```python
from build123d import *

# Parameters (mm, degrees)
F0_R     = 29.0195
F1_DEPTH = 19.05
F2_R     = 2.286
F2_R_2   = 29.0195
F2_R_3   = 21.59
F3_DEPTH = 12.7
F5_DEPTH = 3.175


with BuildPart() as f1:
    # F0 (on Top) → F1 (new body)
    with BuildSketch(Plane.XY):
        with BuildLine():
            Line((58.7375, 1.8415), (58.7375, 93.218))
            ThreePointArc((58.7375, 93.218), (0, 151.9555), (-58.7375, 93.218))
            Line((-58.7375, 93.218), (-58.7375, 1.8415))
            ThreePointArc((-58.7375, 1.8415), (-53.848048, -21.620845), (-39.993711, -41.177066))
            ThreePointArc((-39.993711, -41.177066), (-36.998179, -45.405437), (-35.941, -50.478377))
            Line((-35.941, -50.478377), (-35.941, -74.676))
            ThreePointArc((-35.941, -74.676), (-34.081128, -79.166128), (-29.591, -81.026))
            Line((-29.591, -81.026), (29.591, -81.026))
            ThreePointArc((29.591, -81.026), (34.081128, -79.166128), (35.941, -74.676))
            Line((35.941, -74.676), (35.941, -50.478377))
            ThreePointArc((35.941, -50.478377), (36.998179, -45.405437), (39.993711, -41.177066))
            ThreePointArc((39.993711, -41.177066), (53.848048, -21.620845), (58.7375, 1.8415))
        make_face()
        with BuildLine():
            ThreePointArc((-23.241, -37.899), (-39.933751, -21.065855), (-46.0375, 1.8415))
            Line((-46.0375, 1.8415), (-46.0375, 38.162218))
            ThreePointArc((-46.0375, 38.162218), (-43.247692, 44.89741), (-36.5125, 47.687218))
            Line((-36.5125, 47.687218), (36.5125, 47.687218))
            ThreePointArc((36.5125, 47.687218), (43.247692, 44.89741), (46.0375, 38.162218))
            Line((46.0375, 38.162218), (46.0375, 1.8415))
            ThreePointArc((46.0375, 1.8415), (39.933751, -21.065855), (23.241, -37.899))
            Line((23.241, -37.899), (23.241, -68.326))
            Line((23.241, -68.326), (-23.241, -68.326))
            Line((-23.241, -68.326), (-23.241, -37.899))
        make_face(mode=Mode.SUBTRACT)
        with Locations((0, 93.218)):
            Circle(F0_R, mode=Mode.SUBTRACT)
    extrude(amount=F1_DEPTH)

    # F2 (on face) → F3 (join)
    with BuildSketch(Plane(origin=(0, 0, 0), x_dir=(1, 0, 0), z_dir=(0, 0, -1))):
        with BuildLine():
            ThreePointArc((-58.7375, -93.218), (0, -151.9555), (58.7375, -93.218))
            Line((58.7375, -93.218), (58.7375, -1.8415))
            ThreePointArc((58.7375, -1.8415), (53.848048, 21.620845), (39.993711, 41.177066))
            ThreePointArc((39.993711, 41.177066), (36.998179, 45.405437), (35.941, 50.478377))
            Line((35.941, 50.478377), (35.941, 74.676))
            ThreePointArc((35.941, 74.676), (34.081128, 79.166128), (29.591, 81.026))
            Line((29.591, 81.026), (-29.591, 81.026))
            ThreePointArc((-29.591, 81.026), (-34.081128, 79.166128), (-35.941, 74.676))
            Line((-35.941, 74.676), (-35.941, 50.478377))
            ThreePointArc((-35.941, 50.478377), (-36.998179, 45.405437), (-39.993711, 41.177066))
            ThreePointArc((-39.993711, 41.177066), (-53.848048, 21.620845), (-58.7375, -1.8415))
            Line((-58.7375, -1.8415), (-58.7375, -93.218))
        make_face()
        with Locations((-32.7025, -36.765218)):
            Circle(F2_R, mode=Mode.SUBTRACT)
        with Locations((0, -93.218)):
            Circle(F2_R_2, mode=Mode.SUBTRACT)
        with Locations((32.7025, -36.765218)):
            Circle(F2_R, mode=Mode.SUBTRACT)
        Circle(F2_R_3, mode=Mode.SUBTRACT)
        with Locations((0, 35.56)):
            Circle(F2_R, mode=Mode.SUBTRACT)
    extrude(amount=-F3_DEPTH)

    # F4 (on face) → F5 (cut)
    with BuildSketch(Plane.XY):
        with BuildLine():
            ThreePointArc((-52.3875, 1.8415), (-48.026637, -19.084375), (-35.670066, -36.52641))
            ThreePointArc((-35.670066, -36.52641), (-31.176768, -42.868968), (-29.591, -50.478377))
            Line((-29.591, -50.478377), (-29.591, -74.676))
            Line((-29.591, -74.676), (29.591, -74.676))
            Line((29.591, -74.676), (29.591, -50.478377))
            ThreePointArc((29.591, -50.478377), (31.176768, -42.868968), (35.670066, -36.52641))
            ThreePointArc((35.670066, -36.52641), (48.026637, -19.084375), (52.3875, 1.8415))
            Line((52.3875, 1.8415), (52.3875, 93.218))
            ThreePointArc((52.3875, 93.218), (0, 145.6055), (-52.3875, 93.218))
            Line((-52.3875, 93.218), (-52.3875, 1.8415))
        make_face()
        with BuildLine():
            ThreePointArc((-33.508244, -34.201082), (-45.115932, -17.816141), (-49.2125, 1.8415))
            Line((-49.2125, 1.8415), (-49.2125, 93.218))
            ThreePointArc((-49.2125, 93.218), (0, 142.4305), (49.2125, 93.218))
            Line((49.2125, 93.218), (49.2125, 1.8415))
            ThreePointArc((49.2125, 1.8415), (45.115932, -17.816141), (33.508244, -34.201082))
            ThreePointArc((33.508244, -34.201082), (28.266063, -41.600733), (26.416, -50.478377))
            Line((26.416, -50.478377), (26.416, -71.501))
            Line((26.416, -71.501), (-26.416, -71.501))
            Line((-26.416, -71.501), (-26.416, -50.478377))
            ThreePointArc((-26.416, -50.478377), (-28.266063, -41.600733), (-33.508244, -34.201082))
        make_face(mode=Mode.SUBTRACT)
    extrude(amount=F5_DEPTH, mode=Mode.SUBTRACT)


solid = f1.part
```
The listing builds one solid part. Answer for the finished solid, in the listing's coordinates (mm). A direction names the side the tool comes from. Round coordinates to 2 decimals unless told otherwise and drop trailing zeros. Order: outer loops, then holes, each group sorted by start corner. A loop starts at its lowest first (then second) coordinate and runs counter-clockwise, first axis right, second up. Notation, with made-up numbers: (33.5, -36) - (71.5, -36) arc R15 ccw to (71.5, -13) - close; hole circle Ø7 at (-26.75, 46). An arc over 180 degrees is marked (long way). Put each result on its own line as item: value. Start each with the question number.
(1) For faces 4 (the flat face through (-35.941, -62, 9)), 5 (the cylindrical face through (-48.146, -18.808, 1.565)), 6 (the cylindrical face through (34.031, -79.215, 9.392)), 7 (the flat face through (-23.241, -53, 16)), determine the directions among +Z, -Z, +X, -X, +Y, -Y from which every point of the face is accessible in a straight line to the end or side of a thin tool.
(2) Find section D-D (x = -19). Give the vertices of the cut face in (y, z) (3 decimals).
(3) Find section A-A (x = 0). State how many separate pieces and enclosed holes the cut face has, plus the area to 3 significant figures.
(4) Determine the mould class of faces 1 (the cylindrical face through (1.152, 145.593, 1.565)), 2 (the flat face through (-1, 37, 0)), 3 (the cylindrical face through (1.29, 151.94, 9.39)) for opening direction Y: released by +Y, released by -Y, zero draft, split by the parting line, or undercut.
(5) Straight lines are drawn through the part: probe 1 along X at (y, z) = (-65, 2.5); probe 2 along Y at (x, z) = (0, 4.25); probe 3 along X at (y, z) = (92, 14.5). For each, find the intervals that lie inside material, in ascending order. Write a range as from..to.
(6) Given P1, Ø2.5, axis at y = -65, z = 2.5, coming from the -X side; P2, Ø3, axis at y = -53.5, z = 16.5, coming from the +X side; P3, Ø2, axis at y = -35.5, z = 15.5, coming from the -X side; P4, Ø2.5, axis at x = 32.7, y = 36.77, coming from the +Z side, each flat-ended and moving along its own axis, determine where each tip first touches the part or whether it passes through.
(7) Find section B-B (y = 103). Give the vertices of the cut face in (x, z) (3 decimals), plus the area to 3 significant figures.
Reply:
1. face 4: +Z, -Z, -X, -Y
1. face 5: -Z
1. face 6: +Z, -Z, +X, -Y
1. face 7: +Z
2. outline: (-81.026, 0) - (-74.676, 0) - (-74.676, 3.175) - (-71.501, 3.175) - (-71.501, 0) - (-10.253, 0) - (-10.253, 12.7) - (-68.326, 12.7) - (-68.326, 19.05) - (-81.026, 19.05) - close; (10.253, 0) - (71.283, 0) - (71.283, 19.05) - (47.687, 19.05) - (47.687, 12.7) - (10.253, 12.7) - close; (115.153, 0) - (138.615, 0) - (138.615, 3.175) - (142.039, 3.175) - (142.039, 0) - (148.798, 0) - (148.798, 19.05) - (115.153, 19.05) - close
3. separate pieces: 4
3. enclosed holes: 0
3. area: 1,970 mm^2
4. face 1: undercut
4. face 2: zero draft
4. face 3: released by +Y
5. probe 1: -35.94..-29.59, -26.42..26.42, 29.59..35.94
5. probe 2: -81.03..-37.85, -33.27..-21.59, 21.59..64.2, 122.24..151.96
5. probe 3: -58.74..-28.99, 28.99..58.74
6. P1: x = -35.94
6. P2: x = 35.94
6. P3: x = -46.15
6. P4: through
7. outline: (-57.917, 0) - (-51.466, 0) - (-51.466, 3.175) - (-48.231, 3.175) - (-48.231, 0) - (-27.321, 0) - (-27.321, 19.05) - (-57.917, 19.05) - close; (27.321, 0) - (48.231, 0) - (48.231, 3.175) - (51.466, 3.175) - (51.466, 0) - (57.917, 0) - (57.917, 19.05) - (27.321, 19.05) - close
7. area: 1,150 mm^2
